For this review, use the dimensioned drawing (mm, ordinates from the lowest corner) and the shaded views. Coordinates: 2 decimals unless noted, no trailing zeros. Loops run counter-clockwise (first coordinate to the right, second up) from the corner with the lowest first, then second, coordinate; pieces in that order, holes last.
1. Clearance check with flat-ended pins moving along their axes: P1, Ø0.6, axis at x = 36, z = 14, coming from the +Y side; P2, Ø0.8, axis at x = 31, z = 29.5, coming from the -Y side; P3, Ø0.8, axis at y = 8.5, z = 29.5, coming from the +X side. State where each tip first meets the part, or that it passes through.
2. Mouldability with a two-part tool opening along Y and no side actions: class the marked faces 1, 2, 3 and 4 as pulls with the +Y half, pulls with the -Y half, needs draft (parallel to the pull), parting line crosses it, or undercut.
3. To check wall thickness, follow probe 1 along Y at (x, z) = (30, 7.5); probe 2 along Y at (x, z) = (37.5, 38.5); probe 3 along X at (y, z) = (6.5, 20). State the ranges of each line that lie inside material, in increasing order.
4. Take a section at A-A, the plane z = 15.5. State the section outline as (x, y) points, then the cut area to 3 significant figures.
5. Take a section at B-B, the plane x = 21. State the section outline as (y, z) points.
6. Take a section at C-C, the plane y = 8.25. State the section outline as (x, z) points.
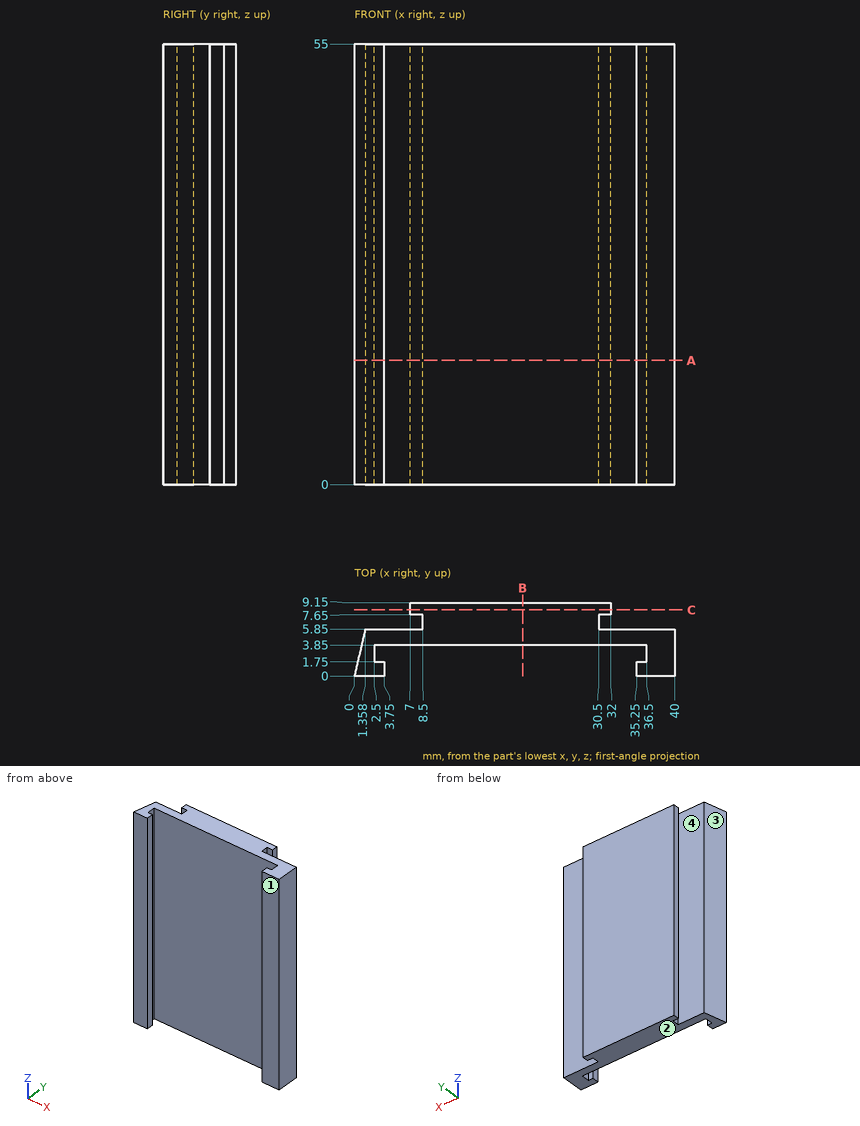
Results list:
1. P1: stops at y = 5.85
1. P2: stops at y = 3.85
1. P3: stops at x = 32
2. face 1: pulls with the -Y half
2. face 2: needs draft
2. face 3: pulls with the +Y half
2. face 4: undercut
3. probe 1: y = 3.85 to 9.15
3. probe 2: y = 0 to 5.85
3. probe 3: x = 8.5 to 30.5
4. outline: (0, 0) - (3.75, 0) - (3.75, 1.75) - (2.5, 1.75) - (2.5, 3.85) - (36.5, 3.85) - (36.5, 1.75) - (35.25, 1.75) - (35.25, 0) - (40, 0) - (40, 5.85) - (30.5, 5.85) - (30.5, 7.65) - (32, 7.65) - (32, 9.15) - (7, 9.15) - (7, 7.65) - (8.5, 7.65) - (8.5, 5.85) - (1.36, 5.85) - close
4. area: 181 mm2
5. outline: (3.85, 0) - (9.15, 0) - (9.15, 55) - (3.85, 55) - close
6. outline: (7, 0) - (32, 0) - (32, 55) - (7, 55) - close
